Geometry: final body of the model. Coordinates: model frame, mm. Face numbers are marked on the shaded views. A direction names the side the tool comes from. Give positions to 0.01 mm unless a question says otherwise; leave off trailing zeros. Write each loop counter-clockwise with the first axis right and the second up, starting at its lowest first coordinate (ties: lowest second). Pieces come first, ordered by that corner, then holes. Notation, with made-up numbers: (-18, 15.5) -> (22, 15.5) arc R13 cw to (22, 25.5) -> close; hole circle Ø3 at (5, 71.5). An arc over 180 degrees is marked (long way). Answer in a Markdown table with one row per item. Add a question column.
from build123d import *

# Parameters (mm, degrees)
SKETCH1_W               = 70.4
SKETCH1_H               = 2
BOSS_EXTRUDE2_DEPTH     = 10
SKETCH2_W               = 2
SKETCH2_H               = 55
BOSS_EXTRUDE3_DEPTH     = 10
SKETCH3_W               = 19
SKETCH3_H               = 3
BOSS_EXTRUDE4_DEPTH     = 2
SKETCH4_W               = 15
SKETCH4_H               = 10
CUT_EXTRUDE2_DEPTH      = 2
SKETCH5_W               = 2
SKETCH5_H               = 3
BOSS_EXTRUDE5_DEPTH     = 1
SKETCH6_W               = 2
SKETCH6_H               = 3
BOSS_EXTRUDE6_DEPTH     = 1
SKETCH7_W               = 57
SKETCH7_H               = 2
BOSS_EXTRUDE7_DEPTH     = 6.6
SKETCH8_W               = 57
SKETCH8_H               = 2
BOSS_EXTRUDE8_DEPTH     = 6.6
BOSS_EXTRUDE9_DEPTH     = 5
SKETCH12_W              = 2
SKETCH12_H              = 5
SKETCH12_H_2            = 40
SKETCH12_H_3            = 30
BOSS_EXTRUDE10_DEPTH    = 20
BOSS_EXTRUDE11_DEPTH    = 3
SKETCH14_W              = 0.5
SKETCH14_H              = 9
CUT_EXTRUDE3_DEPTH      = 3
SKETCH15_W              = 38.4
SKETCH15_H              = 45
CUT_EXTRUDE4_DEPTH      = 3
BOSS_EXTRUDE12_DEPTH    = 0.5
SKETCH17_R              = 1.8
SKETCH17_W              = 3
SKETCH17_H              = 5
CUT_EXTRUDE6_DEPTH      = 3
CUT_EXTRUDE7_DEPTH      = 71
CUT_EXTRUDE7_DEPTH_BACK = 51
SKETCH18_W              = 76.208755975
SKETCH18_H              = 59.797515132
CUT_EXTRUDE8_DEPTH      = 87
CUT_EXTRUDE8_DEPTH_BACK = 25
SKETCH19_W              = 80.230135701
SKETCH19_H              = 33.851054281
SKETCH20_W              = 35
SKETCH20_H              = 3
BOSS_EXTRUDE13_DEPTH    = 2.5
SKETCH21_W              = 2.5
SKETCH21_H              = 35
BOSS_EXTRUDE14_DEPTH    = 8
SKETCH22_R              = 1.8
CUT_EXTRUDE10_DEPTH     = 10


with BuildPart() as part:
    # Sketch1 → Boss-Extrude2 (new body)
    with BuildSketch(Plane(origin=(0, 0, 0), x_dir=(1, 0, 0), z_dir=(0, 1, 0))):
        with Locations((35.2, 1)):
            Rectangle(SKETCH1_W, SKETCH1_H)
    extrude(amount=BOSS_EXTRUDE2_DEPTH)

    # Sketch2 → Boss-Extrude3 (add)
    with BuildSketch(Plane(origin=(0, 10, 0), x_dir=(1, 0, 0), z_dir=(0, 1, 0))):
        with Locations((1, 29.5)):
            Rectangle(SKETCH2_W, SKETCH2_H)
        with Locations((69.4, 29.5)):
            Rectangle(SKETCH2_W, SKETCH2_H)
    extrude(amount=-BOSS_EXTRUDE3_DEPTH)

    # Sketch3 → Boss-Extrude4 (add)
    with BuildSketch(Plane.XY):
        with Locations((35.2, 11.5)):
            Rectangle(SKETCH3_W, SKETCH3_H)
    extrude(amount=-BOSS_EXTRUDE4_DEPTH)

    # Sketch4 → Cut-Extrude2 (cut)
    with BuildSketch(Plane.XY):
        with Locations((35.2, 5)):
            Rectangle(SKETCH4_W, SKETCH4_H)
    extrude(amount=-CUT_EXTRUDE2_DEPTH, mode=Mode.SUBTRACT)

    # Sketch5 → Boss-Extrude5 (add)
    with BuildSketch(Plane.ZY.offset(-25.7)):
        with Locations((-1, 11.5)):
            Rectangle(SKETCH5_W, SKETCH5_H)
    extrude(amount=BOSS_EXTRUDE5_DEPTH)

    # Sketch6 → Boss-Extrude6 (add)
    with BuildSketch(Plane(origin=(44.7, 0, 0), x_dir=(0, 0, -1), z_dir=(1, 0, 0))):
        with Locations((1, 11.5)):
            Rectangle(SKETCH6_W, SKETCH6_H)
    extrude(amount=BOSS_EXTRUDE6_DEPTH)

    # Sketch7 → Boss-Extrude7 (add)
    with BuildSketch(Plane.ZY):
        with Locations((-28.5, 1)):
            Rectangle(SKETCH7_W, SKETCH7_H)
    extrude(amount=BOSS_EXTRUDE7_DEPTH)

    # Sketch8 → Boss-Extrude8 (add)
    with BuildSketch(Plane(origin=(70.4, 0, 0), x_dir=(0, 0, -1), z_dir=(1, 0, 0))):
        with Locations((28.5, 1)):
            Rectangle(SKETCH8_W, SKETCH8_H)
    extrude(amount=BOSS_EXTRUDE8_DEPTH)

    # Sketch10 → Boss-Extrude9 (add)
    with BuildSketch(Plane(origin=(0, 0, -57), x_dir=(-1, 0, 0), z_dir=(0, 0, -1))):
        Polygon((-2, 10), (-2, 0), (6.6, 0), (6.6, 2), (0, 2), (0, 10), align=None)
        Polygon((-77, 0), (-68.4, 0), (-68.4, 10), (-70.4, 10), (-70.4, 2), (-77, 2), align=None)
    extrude(amount=BOSS_EXTRUDE9_DEPTH)

    # Sketch12 → Boss-Extrude10 (add)
    with BuildSketch(Plane(origin=(0, 10, 0), x_dir=(1, 0, 0), z_dir=(0, 1, 0))):
        with Locations((1, 59.5)):
            Rectangle(SKETCH12_W, SKETCH12_H)
        with Locations((1, 37)):
            Rectangle(SKETCH12_W, SKETCH12_H_2)
        with Locations((69.4, 42)):
            Rectangle(SKETCH12_W, SKETCH12_H_3)
        with Locations((69.4, 59.5)):
            Rectangle(SKETCH12_W, SKETCH12_H)
    extrude(amount=BOSS_EXTRUDE10_DEPTH)

    # Sketch13 → Boss-Extrude11 (add)
    with BuildSketch(Plane(origin=(0, 30, 0), x_dir=(1, 0, 0), z_dir=(0, 1, 0))):
        Polygon((0, 17), (35.2, 17), (35.2, 27), (70.4, 27), (70.4, 62), (0, 62), align=None)
    extrude(amount=BOSS_EXTRUDE11_DEPTH)

    # Sketch14 → Cut-Extrude3 (cut)
    with BuildSketch(Plane(origin=(0, 33, 0), x_dir=(1, 0, 0), z_dir=(0, 1, 0))):
        with Locations((11.7, 51)):
            Rectangle(SKETCH14_W, SKETCH14_H)
        with Locations((11.7, 38)):
            Rectangle(SKETCH14_W, SKETCH14_H)
        with Locations((11.7, 25.5)):
            Rectangle(SKETCH14_W, SKETCH14_H)
        with Locations((58.2, 51)):
            Rectangle(SKETCH14_W, SKETCH14_H)
        with Locations((58.2, 38)):
            Rectangle(SKETCH14_W, SKETCH14_H)
    extrude(amount=-CUT_EXTRUDE3_DEPTH, mode=Mode.SUBTRACT)

    # Sketch15 → Cut-Extrude4 (cut)
    with BuildSketch(Plane(origin=(0, 33, 0), x_dir=(1, 0, 0), z_dir=(0, 1, 0))):
        with Locations((35.2, 39.5)):
            Rectangle(SKETCH15_W, SKETCH15_H)
    extrude(amount=-CUT_EXTRUDE4_DEPTH, mode=Mode.SUBTRACT)

    # Sketch16 → Boss-Extrude12 (add)
    with BuildSketch(Plane.XY):
        Polygon((-6.6, 0), (27.7, 0), (27.7, 10), (42.7, 10), (42.7, 0), (77, 0), (77, 2), (70.4, 2), (70.4, 10), (45.7, 10), (45.7, 13), (24.7, 13), (24.7, 10), (0, 10), (0, 2), (-6.6, 2), align=None)
    extrude(amount=BOSS_EXTRUDE12_DEPTH)

    # Sketch17 → Cut-Extrude6 (cut)
    with BuildSketch(Plane(origin=(0, 2, 0), x_dir=(1, 0, 0), z_dir=(0, 1, 0))):
        with Locations(Location((-3.3, 55, 0), (0, 0, 270))):
            Circle(SKETCH17_R)
        with Locations(Location((73.7, 55, 0), (0, 0, 270))):
            Circle(SKETCH17_R)
        with Locations(Location((-3.3, 6.5, 0), (0, 0, 270))):
            Circle(SKETCH17_R)
        with Locations(Location((73.7, 6.5, 0), (0, 0, 270))):
            Circle(SKETCH17_R)
        with Locations(Location((-3.3, 30.75, 0), (0, 0, 270))):
            Circle(SKETCH17_R)
        with Locations(Location((73.7, 30.75, 0), (0, 0, 270))):
            Circle(SKETCH17_R)
        with Locations((-3.3, 14.5)):
            Rectangle(SKETCH17_W, SKETCH17_H)
        with Locations((73.7, 14.5)):
            Rectangle(SKETCH17_W, SKETCH17_H)
    extrude(amount=-CUT_EXTRUDE6_DEPTH, mode=Mode.SUBTRACT)

    # Sketch18 → Cut-Extrude7 (cut, two sides: drawn at the far end of the back side and taken through both)
    with BuildSketch(Plane.ZY.offset(-CUT_EXTRUDE7_DEPTH_BACK)):
        with Locations((-23.895622013, 3.101242434)):
            Rectangle(SKETCH18_W, SKETCH18_H)
    extrude(amount=CUT_EXTRUDE7_DEPTH + CUT_EXTRUDE7_DEPTH_BACK, mode=Mode.SUBTRACT)

    # Sketch19 → Cut-Extrude8 (cut, two sides: drawn at the far end of the back side and taken through both)
    with BuildSketch(Plane.ZY.offset(-68.4).offset(-CUT_EXTRUDE8_DEPTH_BACK)):
        with Locations((-21.88493215, 13.07447286)):
            Rectangle(SKETCH19_W, SKETCH19_H)
    extrude(amount=CUT_EXTRUDE8_DEPTH + CUT_EXTRUDE8_DEPTH_BACK, mode=Mode.SUBTRACT)

    # Sketch20 → Boss-Extrude13 (add)
    with BuildSketch(Plane(origin=(70.4, 0, 0), x_dir=(0, 0, -1), z_dir=(1, 0, 0))):
        with Locations((44.5, 31.5)):
            Rectangle(SKETCH20_W, SKETCH20_H)
    extrude(amount=BOSS_EXTRUDE13_DEPTH)

    # Sketch21 → Boss-Extrude14 (add)
    with BuildSketch(Plane.XZ.offset(-30)):
        with Locations((71.65, -44.5)):
            Rectangle(SKETCH21_W, SKETCH21_H)
    extrude(amount=BOSS_EXTRUDE14_DEPTH)

    # Sketch22 → Cut-Extrude10 (cut)
    with BuildSketch(Plane.ZY.offset(-70.4)):
        with Locations((-52, 26)):
            Circle(SKETCH22_R)
        with Locations((-37, 26)):
            Circle(SKETCH22_R)
    extrude(amount=-CUT_EXTRUDE10_DEPTH, mode=Mode.SUBTRACT)


solid = part.part
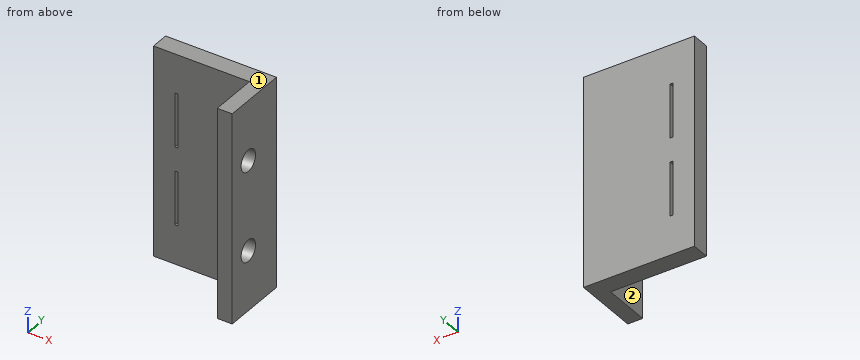
Q1. Line query: probe 1 along X at (y, z) = (32.75, -35); probe 2 along Y at (x, z) = (72.2, -37); probe 3 along X at (y, z) = (28.25, -29). Output: solid intervals per line, ascending. Write a range as from..to.
Q2. Section A-A on y = 26. Return loops of the section in (x, z), and give its area (3 significant figures).
Q3. Section C-C on x = 70.75. Return loops of the section in (y, z), and give its area (3 significant figures).
Q4. Section B-B on z = -34.5. Return loops of the section in (x, y).
Q5. Contact query for flat-ended pins moving along their axis: pin 1 Ø3 at (y, z) = (23.5, -39) entering from -X; pin 2 Ø3 at (x, z) = (67, -41.5) entering from -Y. Output: stop coordinate, or through.
Q6. Section D-D on x = 61.75. Return loops of the section in (y, z).
Q7. Access query for the marked faces 1 and 2. Directions: +Z, -Z, +X, -X, +Y, -Y. A direction counts if a zero-diameter tool reaches every point of the face in a straight line with its end or side. Return the directions, or none.
Checks:
| question | item | result |
|---|---|---|
| 1 | probe 1 | 54.4..57.95, 58.45..72.9 |
| 1 | probe 2 | 22..24.2, 27.8..33 |
| 1 | probe 3 | 70.4..72.9 |
| 2 | outline | (70.4, -62) -> (72.9, -62) -> (72.9, -53.8) -> (70.4, -53.8) -> close; (70.4, -50.2) -> (72.9, -50.2) -> (72.9, -38.8) -> (70.4, -38.8) -> close; (70.4, -35.2) -> (72.9, -35.2) -> (72.9, -27) -> (70.4, -27) -> close |
| 2 | area | 69.5 mm^2 |
| 3 | outline | (22, -62) -> (33, -62) -> (33, -27) -> (22, -27) -> close; hole circle Ø3.6 at (26, -52); hole circle Ø3.6 at (26, -37) |
| 3 | area | 365 mm^2 |
| 4 | outline | (54.4, 30) -> (57.95, 30) -> (57.95, 33) -> (54.4, 33) -> close; (58.45, 30) -> (70.4, 30) -> (70.4, 22) -> (72.9, 22) -> (72.9, 33) -> (58.45, 33) -> close |
| 5 | pin 1 | x = 70.4 |
| 5 | pin 2 | y = 30 |
| 6 | outline | (30, -62) -> (33, -62) -> (33, -27) -> (30, -27) -> close |
| 7 | face 1 | +Z, +X, -X, +Y, -Y |
| 7 | face 2 | +Z, -Z, -X, -Y |
